Autodesk Inventor part; units mm, degrees
ref_plane "YZ Plane" through (0, 0, 0) normal (1, 0, 0) x (0, 1, 0)
ref_plane "XZ Plane" through (0, 0, 0) normal (0, 1, 0) x (-1, 0, 0)
ref_plane "XY Plane" through (0, 0, 0) normal (0, 0, 1) x (1, 0, 0)
sketch "Sketch1" plane through (0, 0, 0) normal (0, 0, 1) x (1, 0, 0)
  line L0 (-12.1708, 16.0073) -> (13.2292, 16.0073)
  line L1 (13.2292, 16.0073) -> (13.2292, -34.7927)
  line L2 (13.2292, -34.7927) -> (-12.1708, -34.7927)
  line L3 (-12.1708, -34.7927) -> (-12.1708, 16.0073)
  line L4 (11.9592, 14.7373) -> (-10.9008, 14.7373)
  line L5 (-10.9008, 14.7373) -> (-10.9008, -33.5227)
  line L6 (-10.9008, -33.5227) -> (11.9592, -33.5227)
  line L7 (11.9592, -33.5227) -> (11.9592, 14.7373)
  point P0 (0, 0)
  dimension "d0" = 25.4
  dimension "d1" = 50.8
  dimension "d2" = 1.27
extrude "Extrusion1" add sketch "Sketch1" along normal blind 146.05
sketch "Sketch2" plane through (-12.1708, 16.0073, 0) normal (0, 1, 0) x (1, 0, 0)
  circle A0 centre (12.7, -12.7) radius 1.7272
  line L0 (25.4, 0) -> (0, 0)
  line L1 (0, 0) -> (0, -146.05)
  point P0 (12.1708, 0)
  dimension "d5" = 3.4544
  dimension "d6" = 12.7
  dimension "d7" = 12.7
extrude "Extrusion2" cut sketch "Sketch2" against normal through all
pattern_linear "Rectangular Pattern1" count 15 spacing 25.4 along (0, 0, 1) of "Extrusion2"
sketch "Sketch5" plane through (-12.1708, -34.7927, 0) normal (-1, 0, 0) x (0, 0, 1)
  line L0 (0, 50.8) -> (0, 0)
  line L1 (95.25, 50.8) -> (146.05, 50.8)
  line L2 (146.05, 50.8) -> (146.05, 203.2)
  line L3 (146.05, 203.2) -> (95.25, 203.2)
  line L4 (95.25, 203.2) -> (95.25, 50.8)
  circle A0 centre (120.65, 101.6) radius 14.2875
  point P0 (0, 34.7927)
  point P1 (120.65, 50.8)
  dimension "d48" = 50.8
  dimension "d49" = 152.4
  dimension "d50" = 28.575
  dimension "d51" = 50.8
sketch "Sketch6" plane through (-12.1708, -34.7927, 0) normal (-1, 0, 0) x (0, 0, 1)
  circle A0 centre (114.3, 25.4) radius 14.2875
  line L0 (146.05, 50.8) -> (146.05, 0)
  point P0 (0, 34.7927)
  point P1 (146.05, 25.4)
  dimension "d52" = 28.575
  dimension "d53" = 31.75
extrude "Extrusion5" cut sketch "Sketch6" against normal blind 25.4
equation "\"d3\" = d13"
equation "\"d10\" = d14"
equation "\"d13\" = 146.05"
equation "\"d14\" = d13"
equation "\"d32\" = 101.6"
properties part number "ElevatorPivotBar1"
Geometry: final body of the model. Coordinates: model frame, mm. A direction names the side the tool comes from. Coordinates: 2 decimals unless noted, no trailing zeros. Order: outer loops, then holes, each group sorted by start corner. A loop starts at its lowest first (then second) coordinate and runs counter-clockwise, first axis right, second up. Notation, with made-up numbers: (-3.75, 74.5) -> (18.25, 74.5) arc R24 ccw to (18.25, 84.5) -> close; hole circle Ø10 at (38.5, -36.75). An arc over 180 degrees is marked (long way). Write each question's results on one line, items separated by ' | '. Start each with the question number.
1) Set-up query: faces 4 (the flat face through (-10.901, -9, 72)), 5 (the flat face through (0, 16.007, 72)). Return all of +Z, -Z, +X, -X, +Y, -Y with unobstructed straight access to the full face (end or side cutting, diameter ignored); none if empty.
2) Cut plane A-A, the plane z = 63.5. Output: boundary loops of the cut face in (x, y), and give its area (3 significant figures).
3) Mould query, pull axis Y, two halves, no side actions, for faces 1 (the cylindrical face through (0.3, -34.15, 10.99)), 2 (the flat face through (1, -34.793, 72)), 3 (the flat face through (0, -33.523, 72)). Classes: released by +Y, released by -Y, zero draft, split by the parting line, or undercut.
4) Cut plane C-C, the plane y = -2. Output: boundary loops of the cut face in (x, z).
5) Cut plane D-D, the plane z = 102.5. Output: boundary loops of the cut face in (x, y).
6) Material intervals for line 1 along Y through (x, z) = (-1, 128); line 2 along X through (y, z) = (-31, 92); line 3 along X through (y, z) = (15.4, 12.7), sorted ascending.
7) First-contact query: pin 1 (3 mm diameter, centred on x = 0.53, z = 88.9, fed in from -Y). Flat tip, straight axial feed; report the tip coordinate or a pass-through.
8) Cut plane B-B, the plane x = -8.25. Output: boundary loops of the cut face in (y, z), and give its area (3 significant figures).
Checks:
1) face 4: +Z, -Z | face 5: +Z, -Z, +X, -X, +Y
2) outline: (-12.17, -34.79) -> (-1.2, -34.79) -> (-1.2, -33.52) -> (-10.9, -33.52) -> (-10.9, 14.74) -> (-1.2, 14.74) -> (-1.2, 16.01) -> (-12.17, 16.01) -> close; (2.26, -34.79) -> (13.23, -34.79) -> (13.23, 16.01) -> (2.26, 16.01) -> (2.26, 14.74) -> (11.96, 14.74) -> (11.96, -33.52) -> (2.26, -33.52) -> close | area: 178 mm^2
3) face 1: zero draft | face 2: released by -Y | face 3: undercut
4) outline: (-12.17, 0) -> (-10.9, 0) -> (-10.9, 102.07) -> (-12.17, 102.07) -> close; (-12.17, 126.53) -> (-10.9, 126.53) -> (-10.9, 146.05) -> (-12.17, 146.05) -> close; (11.96, 0) -> (13.23, 0) -> (13.23, 102.07) -> (11.96, 102.07) -> close; (11.96, 126.53) -> (13.23, 126.53) -> (13.23, 146.05) -> (11.96, 146.05) -> close
5) outline: (-12.17, -34.79) -> (13.23, -34.79) -> (13.23, -17.45) -> (11.96, -17.45) -> (11.96, -33.52) -> (-10.9, -33.52) -> (-10.9, -17.45) -> (-12.17, -17.45) -> close; (-12.17, -1.34) -> (-10.9, -1.34) -> (-10.9, 14.74) -> (11.96, 14.74) -> (11.96, -1.34) -> (13.23, -1.34) -> (13.23, 16.01) -> (-12.17, 16.01) -> close
6) line 1: -34.79 to -33.52, 14.74 to 16.01 | line 2: -12.17 to -10.9, 11.96 to 13.23 | line 3: -12.17 to -1.2, 2.26 to 13.23
7) pin 1: through
8) outline: (-34.79, 0) -> (-33.52, 0) -> (-33.52, 146.05) -> (-34.79, 146.05) -> close; (14.74, 0) -> (16.01, 0) -> (16.01, 146.05) -> (14.74, 146.05) -> close | area: 371 mm^2
